Geometry check sheet. Reference: the model listing, model coordinates, mm. Round coordinates to 2 decimals unless told otherwise and drop trailing zeros. Order: outer loops, then holes, each group sorted by start corner. A loop starts at its lowest first (then second) coordinate and runs counter-clockwise, first axis right, second up. Notation, with made-up numbers: (-8.75, -34) - (40.25, -34) arc R19 ccw to (40.25, -28) - close; hole circle Ø9 at (81, -37). An arc over 180 degrees is marked (long way). Return JSON: item names as keys, results as strings. Group by question number.
Q1. Sectioned sample at A-A, the plane x = 7.5. Record the cut outline in (y, z) (3 decimals), then the cut area to 3 significant figures.
Q2. Material ranges on line 1 along Y through (x, z) = (2, 0); line 2 along X through (y, z) = (0.1, 3); line 3 along Z through (x, y) = (9.5, 0.4) (3 decimals), recorded low to high.
Q3. Sectioned sample at D-D, the plane x = 15.75. Record the cut outline in (y, z).
Q4. Sectioned sample at B-B, the plane z = -1.5. Record the cut outline in (x, y).
Q5. Sectioned sample at C-C, the plane y = 0.3. Record the cut outline in (x, z) (3 decimals).
```python
from build123d import *

# Parameters (mm, degrees)
CROQUIS1_W              = 18
CROQUIS1_H              = 15.7
SALIENTE_EXTRUIR1_DEPTH = 1.5
CROQUIS2_W              = 6.25
CROQUIS2_H              = 6.25
SALIENTE_EXTRUIR2_DEPTH = 0.5


with BuildPart() as part:
    # Croquis1 → Saliente-Extruir1 (new body)
    with BuildSketch(Plane.XZ):
        with Locations((9, 0)):
            Rectangle(CROQUIS1_W, CROQUIS1_H)
    extrude(amount=SALIENTE_EXTRUIR1_DEPTH)

    # Croquis2 → Saliente-Extruir2 (add)
    with BuildSketch(Plane(origin=(0, 0, 0), x_dir=(1, 0, 0), z_dir=(0, 1, 0))):
        with Locations((9.04271605, 0)):
            Rectangle(CROQUIS2_W, CROQUIS2_H)
    extrude(amount=SALIENTE_EXTRUIR2_DEPTH)


solid = part.part
```
Reply:
{
 "1": {"outline": "(-1.5, -7.85) - (0, -7.85) - (0, -3.125) - (0.5, -3.125) - (0.5, 3.125) - (0, 3.125) - (0, 7.85) - (-1.5, 7.85) - close", "area": "26.7 mm^2"},
 "2": {"line 1": "-1.5 to 0", "line 2": "5.92 to 12.17", "line 3": "-3.125 to 3.125"},
 "3": {"outline": "(-1.5, -7.85) - (0, -7.85) - (0, 7.85) - (-1.5, 7.85) - close"},
 "4": {"outline": "(0, -1.5) - (18, -1.5) - (18, 0) - (12.17, 0) - (12.17, 0.5) - (5.92, 0.5) - (5.92, 0) - (0, 0) - close"},
 "5": {"outline": "(5.918, -3.125) - (12.168, -3.125) - (12.168, 3.125) - (5.918, 3.125) - close"}
}
